Autodesk Inventor part; units mm, degrees
ref_plane "YZ Plane" through (0, 0, 0) normal (1, 0, 0) x (0, 1, 0)
ref_plane "XZ Plane" through (0, 0, 0) normal (0, 1, 0) x (-1, 0, 0)
ref_plane "XY Plane" through (0, 0, 0) normal (0, 0, 1) x (1, 0, 0)
sketch "Sketch1" plane through (0, 0, 0) normal (0, 0, 1) x (1, 0, 0)
  line L0 (9.6801, -14.008) -> (7.2052, -11.5331) construction
  line L1 (7.2052, -11.5331) -> (11.5893, -7.1491) construction
  line L2 (11.5893, -7.1491) -> (14.0642, -9.6239) construction
  line L3 (14.0642, -9.6239) -> (9.6801, -14.008) construction
  arc A0 (12.6369, -4.7496) -> (4.7496, -12.6369) centre (0, 0) ccw construction
  line L4 (10.9298, -3.0424) -> (12.6369, -4.7496) construction
  line L5 (11.6618, -4.6122) -> (10.9298, -3.0424) construction
  arc A1 (11.6618, -4.6122) -> (10.8551, -4.47) centre (11.2086, -4.8235) ccw construction
  line L6 (10.7915, -4.5335) -> (10.8551, -4.47) construction
  arc A2 (10.7915, -4.5335) -> (10.6527, -4.9738) centre (11.1451, -4.887) ccw construction
  line L7 (10.915, -6.4612) -> (10.6527, -4.9738) construction
  arc A3 (10.7761, -6.9016) -> (10.915, -6.4612) centre (10.4226, -6.548) ccw construction
  line L8 (6.9016, -10.7761) -> (10.7761, -6.9016) construction
  arc A4 (6.4612, -10.915) -> (6.9016, -10.7761) centre (6.548, -10.4226) ccw construction
  line L9 (6.4612, -10.915) -> (4.9738, -10.6527) construction
  arc A5 (4.9738, -10.6527) -> (4.5335, -10.7915) centre (4.887, -11.1451) ccw construction
  line L10 (4.5335, -10.7915) -> (4.47, -10.8551) construction
  arc A6 (4.47, -10.8551) -> (4.6122, -11.6618) centre (4.8235, -11.2086) ccw construction
  line L11 (4.6122, -11.6618) -> (3.0424, -10.9298) construction
  line L12 (3.0424, -10.9298) -> (4.7496, -12.6369) construction
  line L13 (-1.7167, -14.6498) -> (-1.7167, -17.5) construction
  line L14 (-1.7167, -17.5) -> (1.7167, -17.5) construction
  line L15 (1.7167, -14.6498) -> (1.7167, -17.5) construction
  arc A7 (1.7167, -14.6498) -> (6.9595, -13.0049) centre (0, 0) ccw construction
  arc A8 (6.9595, -13.0049) -> (8.2728, -15.1789) centre (8.2994, -13.6792) ccw construction
  line L16 (8.2728, -15.1789) -> (7.6816, -15.1684) construction
  arc A9 (8.5249, -17.8901) -> (7.6816, -15.1684) centre (7.655, -16.6682) ccw construction
  line L17 (8.5249, -17.8901) -> (13.5161, -14.3366) construction
  line L18 (13.5161, -14.3366) -> (13.5161, -12.2823) construction
  line L19 (13.5161, -12.2823) -> (14.6168, -12.2823) construction
  line L20 (14.6168, -12.2823) -> (14.6168, -1.9776) construction
  arc A10 (14.6168, -1.9776) -> (1.7167, 14.6498) centre (0, 0) ccw construction
  line L21 (1.7167, 14.6498) -> (1.7167, 17.5) construction
  line L22 (-1.7167, 17.5) -> (1.7167, 17.5) construction
  line L23 (-1.7167, 14.6498) -> (-1.7167, 17.5) construction
  arc A11 (-1.7167, 14.6498) -> (-14.2817, -3.6872) centre (0, 0) ccw construction
  line L24 (-14.2817, -3.6872) -> (-15.4135, -5.7935) construction
  arc A12 (-15.4135, -5.7935) -> (-14.5984, -8.502) centre (-13.6517, -6.7402) ccw construction
  line L25 (-14.5984, -8.502) -> (-9.6326, -11.1703) construction
  arc A13 (-9.6326, -11.1703) -> (-1.7167, -14.6498) centre (0, 0) ccw construction
  line L26 (-24.6, 24.6) -> (25.2, -25.2) construction
  line L27 (25.2, 24.6) -> (-24.6, -25.2) construction
  arc A14 (-3.041, 10.05) -> (-10.224, -2.3914) centre (0, 0) ccw
  circle A15 centre (0, 0) radius 10.1 construction
  line L28 (-3.041, 10.05) -> (3.041, 10.05)
  line L29 (-7.1831, -7.6586) -> (-10.224, -2.3914)
  line L30 (10.224, -2.3914) -> (7.1831, -7.6586)
  arc A16 (3.041, 10.05) -> (-3.041, 10.05) centre (0, 0) ccw
  arc A17 (10.224, -2.3914) -> (3.041, 10.05) centre (0, 0) ccw
  arc A18 (7.1831, -7.6586) -> (10.224, -2.3914) centre (0, 0) ccw
  arc A19 (-7.1831, -7.6586) -> (7.1831, -7.6586) centre (0, 0) ccw
  arc A20 (-10.224, -2.3914) -> (-7.1831, -7.6586) centre (0, 0) ccw
  arc A21 (10.7054, -6.8309) -> (10.8165, -6.4786) centre (10.4226, -6.548) ccw
  line L31 (10.8165, -6.4786) -> (10.5542, -4.9912)
  arc A22 (10.7208, -4.4628) -> (10.5956, -4.6461) centre (11.1451, -4.887) ccw construction
  line L32 (10.7208, -4.4628) -> (10.7844, -4.3992) construction
  arc A23 (11.7601, -5.0598) -> (10.7844, -4.3992) centre (11.2086, -4.8235) ccw construction
  line L33 (11.7601, -5.0598) -> (10.5994, -2.5707) construction
  line L34 (10.5994, -2.5707) -> (12.5972, -4.5684) construction
  arc A24 (12.5972, -4.5684) -> (4.5684, -12.5972) centre (0, 0) ccw construction
  line L35 (4.5684, -12.5972) -> (2.5707, -10.5994) construction
  line L36 (2.5707, -10.5994) -> (4.2491, -11.3821) construction
  arc A25 (4.3992, -10.7844) -> (4.2491, -11.3821) centre (4.8235, -11.2086) ccw construction
  line L37 (4.3992, -10.7844) -> (4.4628, -10.7208) construction
  arc A26 (4.9912, -10.5542) -> (4.6461, -10.5956) centre (4.887, -11.1451) ccw
  line L38 (4.9912, -10.5542) -> (6.4786, -10.8165)
  arc A27 (6.4786, -10.8165) -> (6.8309, -10.7054) centre (6.548, -10.4226) ccw
  line L39 (6.8309, -10.7054) -> (10.7054, -6.8309)
  circle A28 centre (0, 0) radius 11.5695
  arc A29 (4.6461, -10.5956) -> (4.4628, -10.7208) centre (4.887, -11.1451) ccw construction
  arc A30 (10.5956, -4.6461) -> (10.5542, -4.9912) centre (11.1451, -4.887) ccw
  dimension "d4" = 20.2
  dimension "d5" = 10.05
  dimension "d6" = 21
  dimension "d9" = 360
  dimension "d11" = 0.1
extrude "Extrusion1" add sketch "Sketch1" against normal blind 5 contours A16 L28 | L29 A20 | A18 L30 | L39 A27 L38 A26 A28 A30 L31 A21 | A28
sketch "Sketch3" plane through (0, 0, -5) normal (0, 0, -1) x (-1, 0, 0)
  line L0 (10.224, -2.3914) -> (7.1831, -7.6586)
  arc A0 (-7.1831, -7.6586) -> (7.1831, -7.6586) centre (0, 0) ccw
  line L1 (-7.1831, -7.6586) -> (-10.224, -2.3914)
  arc A1 (-3.041, 10.05) -> (-10.224, -2.3914) centre (0, 0) ccw
  line L2 (-3.041, 10.05) -> (3.041, 10.05)
  arc A2 (10.224, -2.3914) -> (3.041, 10.05) centre (0, 0) ccw
  arc A3 (-10.8165, -6.4786) -> (-10.7054, -6.8309) centre (-10.4226, -6.548) ccw
  line L3 (-10.7054, -6.8309) -> (-6.8309, -10.7054)
  arc A4 (-6.8309, -10.7054) -> (-6.4786, -10.8165) centre (-6.548, -10.4226) ccw
  line L4 (-6.4786, -10.8165) -> (-4.9912, -10.5542)
  arc A5 (-4.6461, -10.5956) -> (-4.9912, -10.5542) centre (-4.887, -11.1451) ccw
  arc A6 (-4.6461, -10.5956) -> (-10.5956, -4.6461) centre (0, 0) ccw
  arc A7 (-10.5542, -4.9912) -> (-10.5956, -4.6461) centre (-11.1451, -4.887) ccw
  line L5 (-10.5542, -4.9912) -> (-10.8165, -6.4786)
  circle A8 centre (0, 0) radius 8
  circle A9 centre (0, 0) radius 10.5
  dimension "d17" = 16
extrude "Extrusion3" add sketch "Sketch3" along normal blind 8.5 contours A9 L0 | L0 A0 L1 A1 L2 A2 | A9 L1 | L2 A9 | L5 A7 A6 A5 L4 A4 L3 A3
sketch "Sketch4" plane through (6.8309, -10.7054, 0) normal (0.7071, -0.7071, 0) x (0, 0, -1)
  line L0 (0, 0) -> (0, 5.4794) construction
  line L1 (0, 0) -> (13.5, 0) construction
  line L2 (13.5, 5.4794) -> (13.5, 0) construction
  line L3 (0, 5.4794) -> (13.5, 5.4794) construction
  line L4 (0, 2.7397) -> (13.5, 2.7397) construction
  circle A0 centre (11.9, 2.7397) radius 1.4
  circle A1 centre (6.54, 2.7397) radius 1.4
  dimension "d20" = 2.8
  dimension "d21" = 1.6
  dimension "d47" = 2.8
  dimension "d48" = 5.36
extrude "Extrusion4" cut sketch "Sketch4" against normal up to surface
properties part number "20_focus_inlet_linearflexure_objective_mount_v0"
Work out the finished part from the listing and answer in its coordinate system (mm). A direction names the side the tool comes from. Round coordinates to 2 decimals unless told otherwise and drop trailing zeros. Write each loop counter-clockwise with the first axis right and the second up, starting at its lowest first coordinate (ties: lowest second). Pieces come first, ordered by that corner, then holes. Notation, with made-up numbers: M 13.5,0.5 L 60.5,0.5 A12 ccw 60.5,13.5 Z; hole C 48,39.5 d11. An arc over 180 degrees is marked long. Use a Markdown table: item, result.
1) The part is cut by section A-A on z = -8.5. Give the vertices of the cut face in (x, y), plus the area to 3 significant figures.
Taken from the geometry:
| item | result |
|---|---|
| outline | M 4.65,-10.6 A0.6 cw 4.99,-10.55 L 6.48,-10.82 A0.4 ccw 6.83,-10.71 L 10.71,-6.83 A0.4 ccw 10.82,-6.48 L 10.55,-4.99 A0.6 cw 10.6,-4.65 A11.57 ccw long Z; hole C 0,0 d16 |
| area | 226 mm2 |
2) Which of the six approach directions +Z, -Z, +X, -X, +Y, -Y give full straight-line access (tool end or side, diameter ignored) to faces 4 (the face through (10.69, -5.75, -6.66)), 5 (the face through (-8.682, -5.062, -2.465)), 6 (the face through (5.724, -10.684, -6.656)), 7 (the face through (-7.86, 8.49, -9.19))?
Taken from the geometry:
| item | result |
|---|---|
| face 4 | +Z, -Z, +X |
| face 5 | +Z |
| face 6 | +Z, -Z, -Y |
| face 7 | +Z, -Z |
3) Consider line 1 (Y direction, x = 0, z = -9.5); line 2 (Z direction, x = 2.75, y = 9.25); line 3 (Y direction, x = -6.5, z = -1.5). Determine where each line is inside the solid, lowest interval first. Write a range as [from, to].
Taken from the geometry:
| item | result |
|---|---|
| line 1 | y = [-11.57, -8], [8, 11.57] |
| line 2 | z = [-13.5, -5] |
| line 3 | y = [-9.57, -8.25], [8.25, 9.57] |
4) Determine the mould class of faces 1 (the face through (3, -8, -13.5)), 2 (the face through (-9.037, 5.346, -2.465)), 3 (the face through (7.489, -6.894, -13.235)) for opening direction Z: pulls with the +Z half, pulls with the -Z half, needs draft (parallel to the pull), parting line crosses it, or undercut.
Taken from the geometry:
| item | result |
|---|---|
| face 1 | pulls with the -Z half |
| face 2 | needs draft |
| face 3 | undercut |
5) Flat-ended cylindrical pins translate along their axes: pin 1 (2 mm diameter, centred on x = -7, z = -7, fed in from +Y); pin 2 (5.5 mm diameter, centred on x = -1, z = -1.5, fed in from -Y); pin 3 (10.5 mm diameter, centred on x = -1.5, y = 3, fed in from +Z); pin 4 (8 mm diameter, centred on y = 6.5, z = -4, fed in from +X). Find the tip coordinate at first contact, or state that the pin passes through.
Taken from the geometry:
| item | result |
|---|---|
| pin 1 | stops at y = 9.89 |
| pin 2 | stops at y = -11.57 |
| pin 3 | stops at z = -5 |
| pin 4 | stops at x = 11.3 |
